```python
from build123d import *

# Parameters (mm, degrees)
SKETCH1_R           = 5.5
BOSS_EXTRUDE1_DEPTH = 3
MOVE_START          = -3
MOVE_FACE1_DEPTH    = 6
SKETCH3_R           = 17.792629247
SKETCH3_R_2         = 4.75
BOSS_EXTRUDE3_DEPTH = 6
FILLET3_R           = 147
FILLET4_R           = 10
SKETCH5_W           = 25
SKETCH5_H           = 6
SKETCH5_W_2         = 20
CUT_EXTRUDE1_DEPTH  = 123.739451528
MOVE_FACE2_DEPTH    = 6
FILLET5_R           = 5


with BuildPart() as part:
    # Sketch1 → Boss-Extrude1 (new, symmetric)
    with BuildSketch(Plane.XY):
        with BuildLine():
            Line((100.725085642, 12), (-7.531031869, 22.507881701))
            Line((-7.531031869, 22.507881701), (0, 0))
            Line((0, 0), (2.007571917, -6))
            Line((2.007571917, -6), (88.851239866, -6))
            ThreePointArc((88.851239866, -6), (98.632352269, -18.710186538), (113.423722773, -12.510641371))
            ThreePointArc((113.423722773, -12.510641371), (113.737903109, 3.196949424), (100.725085642, 12))
        make_face()
        with Locations((102, -6)):
            Circle(SKETCH1_R, mode=Mode.SUBTRACT)
    extrude(amount=BOSS_EXTRUDE1_DEPTH, both=True)

    # Move Face1: read off the stored shape, not the designer's step
    # Move Face1 outline → Move Face1 (add)
    with BuildSketch(Plane.XY.offset(MOVE_START)):
        Polygon((-7.531031869, 22.5078817), (-44.042319528, 26.051850395), (-33.317920404, -6), (2.007571917, -6), align=None)
    extrude(amount=MOVE_FACE1_DEPTH)

    # Sketch3 → Boss-Extrude3 (add)
    with BuildSketch(Plane.XY.offset(3)):
        with Locations((102, -6)):
            Circle(SKETCH3_R)
        with Locations((102, -6)):
            Circle(SKETCH3_R_2, mode=Mode.SUBTRACT)
    extrude(amount=-BOSS_EXTRUDE3_DEPTH)

    # Fillet3
    fillet3_edges = [part.edges().sort_by_distance(p)[0] for p in [
        (102.186094391, 11.791656034, 0),
    ]]
    fillet(fillet3_edges, radius=FILLET3_R)

    # Fillet4
    fillet4_edges = [part.edges().sort_by_distance(p)[0] for p in [
        (84.207370753, -6, 0),
    ]]
    fillet(fillet4_edges, radius=FILLET4_R)

    # Sketch5 → Cut-Extrude1 (cut, through all)
    with BuildSketch(Plane(origin=(0, 0, -3), x_dir=(-1, 0, 0), z_dir=(0, 0, -1))):
        with Locations((37.25, -3)):
            Rectangle(SKETCH5_W, SKETCH5_H)
        with Locations((-21.983719278, -3)):
            Rectangle(SKETCH5_W_2, SKETCH5_H)
    extrude(amount=-CUT_EXTRUDE1_DEPTH, mode=Mode.SUBTRACT)

    # Move Face2: read off the stored shape, not the designer's step
    # Move Face2 outline → Move Face2 (add)
    with BuildSketch(Plane.XY.offset(MOVE_START)):
        Polygon((-44.569041147, 26.102976637), (-35.325492321, 0), (-44.042319528, 26.051850395), align=None)
    extrude(amount=MOVE_FACE2_DEPTH)

    # Fillet5
    fillet5_edges = [part.edges().sort_by_distance(p)[0] for p in [
        (-35.325492321, 0, 0),
    ]]
    fillet(fillet5_edges, radius=FILLET5_R)


solid = part.part
```
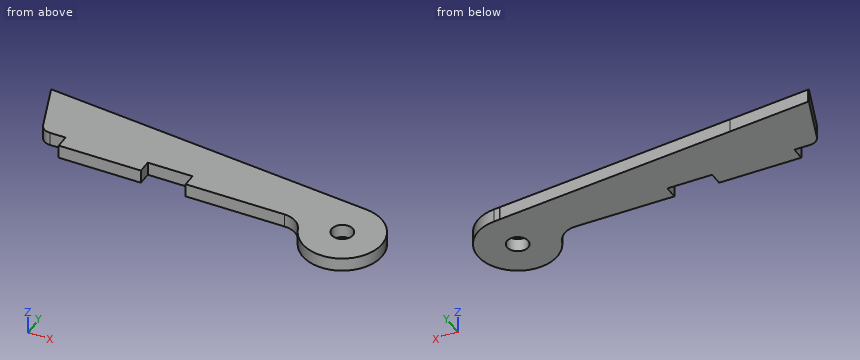
Could you check a few things on this model? Use its own coordinates, in mm. Coordinates: 2 decimals unless noted, no trailing zeros. Loops run counter-clockwise (first coordinate to the right, second up) from the corner with the lowest first, then second, coordinate; pieces in that order, holes last. Notation, with made-up numbers: M -29,4.25 L 3,4.25 A20 ccw 3,30.25 Z; hole C 38.5,34 d5. An arc over 180 degrees is marked long. Put each result on its own line as item: value. Start each with the question number.
(1) I need wall thicknesses on line 1 (X direction, y = -9, z = -2.5); line 2 (Y direction, x = 102, z = 0.55); line 3 (X direction, y = -8, z = -1.25). Which ranges of each line are inside material? Lowest first, please. Write a range as from..to.
(2) Suppose I cut it at B-B on x = -0.5. Please give me the cut outline in (y, z), then the cut area to 3 significant figures.
(3) Will these pins go through, and if not, where does the flat tip stop? P1, Ø3, axis at y = -2, z = 1, coming from the -X side; P2, Ø1.5, axis at x = -0.5, z = 0, coming from the -Y side; P3, Ø1.8, axis at x = 19, z = 1, coming from the -Y side; P4, Ø4, axis at x = 47.5, y = 18, coming from the -Z side.
(4) Suppose I cut it at A-A on x = 67. Please give me the cut outline in (y, z).
Solutions:
1. line 1: x = 83.21..98.32, 105.68..119.54
1. line 2: y = -23.79..-10.75, -1.25..11.87
1. line 3: x = 82.07..97.69, 106.31..119.68
2. outline: M -6,-3 L 21.83,-3 L 21.83,3 L -6,3 Z
2. area: 167 mm2
3. P1: stops at x = -24.75
3. P2: stops at y = -6
3. P3: stops at y = 0
3. P4: stops at z = -3
4. outline: M -6,-3 L 15.27,-3 L 15.27,3 L -6,3 Z
